Part model, mm, in its own coordinate system. Face numbers are marked on the shaded views. A direction names the side the tool comes from. Round coordinates to 2 decimals unless told otherwise and drop trailing zeros. Loops run counter-clockwise (first coordinate to the right, second up) from the corner with the lowest first, then second, coordinate; pieces in that order, holes last.
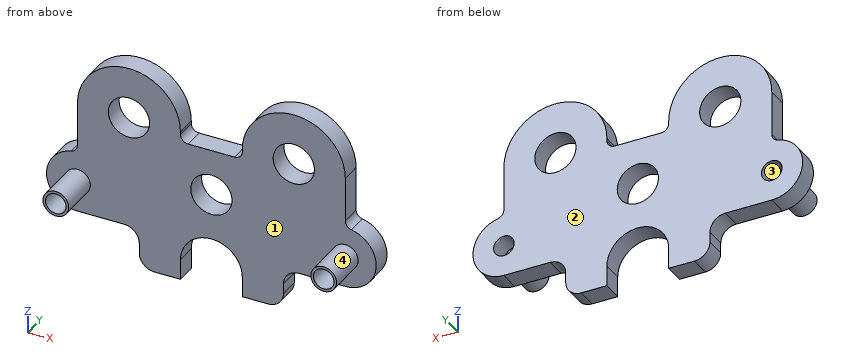
from build123d import *

# Parameters (mm, degrees)
F0_R     = 7.9375
F0_R_2   = 12.7
F0_R_3   = 6.35
F1_DEPTH = 12.7
F2_DEPTH = 25.4


with BuildPart() as f1:
    # F0 (on Front) → F1 (new body)
    with BuildSketch(Plane.XZ):
        with BuildLine():
            Line((14.2875, 28.575), (0, 28.575))
            Line((0, 28.575), (-14.2875, 28.575))
            ThreePointArc((-14.2875, 28.575), (-17.655096, 29.969904), (-19.05, 33.3375))
            Line((-19.05, 33.3375), (-19.05, 34.925))
            ThreePointArc((-19.05, 34.925), (-50.8, 66.675), (-82.55, 34.925))
            Line((-82.55, 34.925), (-82.55, 7.45639))
            ThreePointArc((-82.55, 7.45639), (-83.623483, 4.44432), (-86.36, 2.790112))
            ThreePointArc((-86.36, 2.790112), (-101.503534, -17.789696), (-82.55, -34.925))
            Line((-82.55, -34.925), (-53.975, -34.925))
            ThreePointArc((-53.975, -34.925), (-47.239808, -37.714808), (-44.45, -44.45))
            Line((-44.45, -44.45), (-44.45, -50.8))
            ThreePointArc((-44.45, -50.8), (-41.660192, -57.535192), (-34.925, -60.325))
            Line((-34.925, -60.325), (-19.05, -60.325))
            Line((-19.05, -60.325), (-19.05, -47.625))
            ThreePointArc((-19.05, -47.625), (0, -28.575), (19.05, -47.625))
            Line((19.05, -47.625), (19.05, -60.325))
            Line((19.05, -60.325), (34.925, -60.325))
            ThreePointArc((34.925, -60.325), (41.660192, -57.535192), (44.45, -50.8))
            Line((44.45, -50.8), (44.45, -44.45))
            ThreePointArc((44.45, -44.45), (47.239808, -37.714808), (53.975, -34.925))
            Line((53.975, -34.925), (82.55, -34.925))
            ThreePointArc((82.55, -34.925), (101.503534, -17.789696), (86.36, 2.790112))
            ThreePointArc((86.36, 2.790112), (83.623483, 4.44432), (82.55, 7.45639))
            Line((82.55, 7.45639), (82.55, 34.925))
            ThreePointArc((82.55, 34.925), (50.8, 66.675), (19.05, 34.925))
            Line((19.05, 34.925), (19.05, 33.3375))
            ThreePointArc((19.05, 33.3375), (17.655096, 29.969904), (14.2875, 28.575))
        make_face()
        with Locations((-82.55, -15.875)):
            Circle(F0_R, mode=Mode.SUBTRACT)
        Circle(F0_R_2, mode=Mode.SUBTRACT)
        with Locations((82.55, -15.875)):
            Circle(F0_R, mode=Mode.SUBTRACT)
        with Locations((-50.8, 34.925)):
            Circle(F0_R_2, mode=Mode.SUBTRACT)
        with Locations((50.8, 34.925)):
            Circle(F0_R_2, mode=Mode.SUBTRACT)
        with Locations((82.55, -15.875)):
            Circle(F0_R)
        with Locations((82.55, -15.875)):
            Circle(F0_R_3, mode=Mode.SUBTRACT)
        with Locations((-82.55, -15.875)):
            Circle(F0_R)
        with Locations((-82.55, -15.875)):
            Circle(F0_R_3, mode=Mode.SUBTRACT)
    extrude(amount=-F1_DEPTH)

    # F0 (on Front) → F2 (join)
    with BuildSketch(Plane.XZ):
        with Locations((-82.55, -15.875)):
            Circle(F0_R)
        with Locations((-82.55, -15.875)):
            Circle(F0_R_3, mode=Mode.SUBTRACT)
        with Locations((82.55, -15.875)):
            Circle(F0_R)
        with Locations((82.55, -15.875)):
            Circle(F0_R_3, mode=Mode.SUBTRACT)
    extrude(amount=F2_DEPTH)


solid = f1.part
1) Drop flat-ended pins along their axis: pin 1 Ø5 at (y, z) = (5.5, -47.5) entering from -X; pin 2 Ø10 at (x, z) = (52, 52) entering from -Y; pin 3 Ø3 at (y, z) = (6.5, -46.5) entering from +X; pin 4 Ø20.5 at (x, z) = (0, 0) entering from +Y. Give the stop position or say it passes through.
Values:
pin 1: stops at x = -44.45
pin 2: stops at y = 0
pin 3: stops at x = 44.45
pin 4: passes through
2) Slice it at A-A, the plane x = 0. Give the cut face in (y, z) (3 decimals), then the cut area to 3 significant figures.
Values:
outline: (0, -28.575) - (12.7, -28.575) - (12.7, -12.7) - (0, -12.7) - close; (0, 12.7) - (12.7, 12.7) - (12.7, 28.575) - (0, 28.575) - close
area: 403 mm2
3) Tool access for the marked faces 3 and 4: list every direction of +Z, -Z, +X, -X, +Y, -Y with a clear straight run to the whole face (end or side of a thin tool).
Values:
face 3: +Y, -Y
face 4: -Y
4) Wall check: line 1 along X through (y, z) = (-5, -20.5); line 2 along Y through (x, z) = (-42, -33.5); line 3 along X through (y, z) = (-14, -12). Give the ranges that are in metal, low to high.
Values:
line 1: x = -89 to -86.9, -78.2 to -76.1, 76.1 to 78.2, 86.9 to 89
line 2: y = 0 to 12.7
line 3: x = -89.48 to -87.58, -77.52 to -75.62, 75.62 to 77.52, 87.58 to 89.48
5) Slice it at B-B, the plane z = -41. Give the cut face in (x, y).
Values:
outline: (-45.1, 0) - (-17.86, 0) - (-17.86, 12.7) - (-45.1, 12.7) - close; (17.86, 0) - (45.1, 0) - (45.1, 12.7) - (17.86, 12.7) - close
6) Mould opens along X. For the marked faces 1 and 2 say: released by +X, released by -X, zero draft, split by the parting line, or undercut.
Values:
face 1: undercut
face 2: zero draft
7) Slice it at C-C, the plane y = -15.5. Give the number of separate pieces and of enclosed holes in the cut face, then the cut area to 3 significant figures.
Values:
separate pieces: 2
enclosed holes: 2
area: 143 mm2
